The model under review builds one solid part; all positions refer to its coordinate system, in mm. A direction names the side the tool comes from. Coordinates: 2 decimals unless noted, no trailing zeros. Order: outer loops, then holes, each group sorted by start corner. A loop starts at its lowest first (then second) coordinate and runs counter-clockwise, first axis right, second up.
Autodesk Inventor part; units mm, degrees
ref_plane "YZ Plane" through (0, 0, 0) normal (1, 0, 0) x (0, 1, 0)
ref_plane "XZ Plane" through (0, 0, 0) normal (0, 1, 0) x (-1, 0, 0)
ref_plane "XY Plane" through (0, 0, 0) normal (0, 0, 1) x (1, 0, 0)
sketch "Sketch1" plane through (0, 0, 0) normal (0, 0, 1) x (1, 0, 0)
  line L0 (0, 0) -> (45, 0)
  line L1 (45, 0) -> (45, -20)
  line L2 (45, -20) -> (0, -20)
  line L3 (0, -20) -> (0, 0)
  dimension "d0" = 45
  dimension "d1" = 20
extrude "Extrusion1" add sketch "Sketch1" along normal blind 1
sketch "Sketch2" plane through (0, 0, 1) normal (0, 0, 1) x (1, 0, 0)
  circle A0 centre (9.5, -10) radius 8
  circle A1 centre (35.5, -10) radius 8
  line L0 (0, -20) -> (45, -20)
  line L1 (0, 0) -> (0, -20)
  dimension "d4" = 16
  dimension "d5" = 16
  dimension "d6" = 26
  dimension "d7" = 10
  dimension "d8" = 9.5
extrude "Extrusion2" add sketch "Sketch2" along normal blind 12
sketch "Sketch3" plane through (0, 0, 1) normal (0, 0, 1) x (1, 0, 0)
  line L0 (17.5, -0.5) -> (27.5, -0.5)
  line L1 (27.5, -0.5) -> (27.5, -5.5)
  line L2 (27.5, -5.5) -> (17.5, -5.5)
  line L3 (17.5, -5.5) -> (17.5, -0.5)
  line L4 (0, 0) -> (0, -20)
  line L5 (45, 0) -> (0, 0)
  dimension "d11" = 10
  dimension "d12" = 5
  dimension "d13" = 17.5
  dimension "d14" = 0.5
extrude "Extrusion3" add sketch "Sketch3" along normal blind 3
fillet "Fillet1" radius 2 4 edges at (27.5, -0.5, 2.5) (27.5, -5.5, 2.5) (17.5, -0.5, 2.5) (17.5, -5.5, 2.5)
fillet "Fillet2" radius 0.5 8 edges at (17.5, -3, 4) (18.0858, -1.0858, 4) (22.5, -0.5, 4) (26.9142, -1.0858, 4) (27.5, -3, 4) (26.9142, -4.9142, 4) (22.5, -5.5, 4) (18.0858, -4.9142, 4)
sketch "Sketch4" plane through (0, 0, 0) normal (0, 0, -1) x (-1, 0, 0)
  point P0 (0, 0)
sketch "Sketch5" plane through (0, 0, 0) normal (0, 0, -1) x (-1, 0, 0)
  line L0 (0, -20) -> (-45, -20)
  line L1 (-27.5, -19.5) -> (-17.5, -19.5)
  line L2 (-17.5, -19.5) -> (-17.5, -17)
  line L3 (-17.5, -17) -> (-27.5, -17)
  line L4 (-27.5, -17) -> (-27.5, -19.5)
  line L5 (-45, -20) -> (-45, 0)
  point P0 (0, 0)
  point P1 (-17.5, -18.25)
  point P2 (-27.5, -18.25)
  point P3 (-17.5, -20)
  dimension "d20" = 10
  dimension "d21" = 17.5
  dimension "d24" = 0.5
  dimension "d25" = 2.5
extrude "Extrusion4" add sketch "Sketch5" along normal blind 10
properties part number "UltrasonicSensor"
(1) Machinability: for faces 5 (the face through (22, -3, 4)), 6 (the face through (7.77, -2.19, 6.92)), 7 (the face through (22, -0.5, 2)), 8 (the face through (17.5, -3, 2)), 9 (the face through (17.5, -18, -5)), which of the approach directions +Z, -Z, +X, -X, +Y, -Y give a long, thin tool a straight path to every point of the face, cutting with its end or side? Answer none if there is none.
A:
face 5: +Z, +Y, -Y
face 6: +Z
face 7: +Z, +X, -X, +Y
face 8: +Z, +Y
face 9: -Z, -X, +Y, -Y
(2) Wall thickness on probe 1 along X at (y, z) = (-15.25, 2.75); probe 2 along Z at (x, y) = (9, -2.25); probe 3 along X at (y, z) = (-6.5, 3.5): over which ranges is each line inside the solid? List them lowest first.
A:
probe 1: x = 3.46 to 15.54, 29.46 to 41.54
probe 2: z = 0 to 13
probe 3: x = 2.31 to 16.69, 28.31 to 42.69
(3) For pin 1 Ø3 at (y, z) = (-18, -4.5) entering from -X; pin 2 Ø10 at (y, z) = (-4.5, 7.5) entering from -X; pin 3 Ø3 at (x, z) = (20.5, -5) entering from +Y; pin 4 Ø8 at (y, z) = (-7, 1.5) entering from -X, all flat-tipped, find the tip position at first contact; note any pin that passes through.
A:
pin 1: stops at x = 17.5
pin 2: stops at x = 1.52
pin 3: stops at y = -17
pin 4: stops at x = 0
(4) We need section D-D, the plane x = 38.5. Write out the cut boundary in (y, z), and give its area (3 significant figures).
A:
outline: (-20, 0) - (0, 0) - (0, 1) - (-2.58, 1) - (-2.58, 13) - (-17.42, 13) - (-17.42, 1) - (-20, 1) - close
area: 198 mm2
(5) Draft analysis for pull direction X (two halves, no side actions). For faces 1 (the face through (23, -19.5, -5)), 2 (the face through (27.5, -18, -5)), 3 (the face through (0, -10.1, 0.5)), 4 (the face through (22, -10, 1)), state which applies: released by +X, released by -X, zero draft, split by the parting line, or undercut.
A:
face 1: zero draft
face 2: released by +X
face 3: released by -X
face 4: undercut
(6) We need section B-B, the plane y = -10. Write out the cut boundary in (x, z).
A:
outline: (0, 0) - (45, 0) - (45, 1) - (43.5, 1) - (43.5, 13) - (27.5, 13) - (27.5, 1) - (17.5, 1) - (17.5, 13) - (1.5, 13) - (1.5, 1) - (0, 1) - close
(7) We need section A-A, the plane x = 20.5. Write out the cut boundary in (y, z).
A:
outline: (-20, 0) - (-19.5, 0) - (-19.5, -10) - (-17, -10) - (-17, 0) - (0, 0) - (0, 1) - (-0.5, 1) - (-0.5, 3.5) arc R0.5 ccw to (-1, 4) - (-5, 4) arc R0.5 ccw to (-5.5, 3.5) - (-5.5, 1) - (-20, 1) - close
(8) We need section C-C, the plane z = 7. Write out the cut boundary in (x, y), and give its area (3 significant figures).
A:
outline: circle Ø16 at (9.5, -10); circle Ø16 at (35.5, -10)
area: 402 mm2
